The model under review builds one solid part; all positions refer to its coordinate system, in mm. Face numbers are marked on the shaded views. A direction names the side the tool comes from. Round coordinates to 2 decimals unless told otherwise and drop trailing zeros. Loops run counter-clockwise (first coordinate to the right, second up) from the corner with the lowest first, then second, coordinate; pieces in that order, holes last. Notation, with made-up numbers: (-16, 26) -> (36, 26) arc R14 cw to (36, 46) -> close; hole circle Ø4 at (82, 4). An arc over 180 degrees is marked (long way). Use CSV: the item, a comma, the result in double quotes. Start each with the question number.
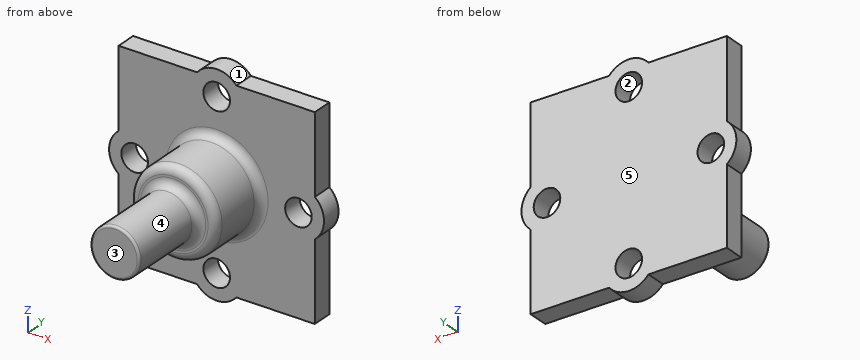
```python
from build123d import *

# Parameters (mm, degrees)
SKETCH1_R           = 3.25
BOSS_EXTRUDE1_DEPTH = 5
SKETCH2_W           = 32.64938716
SKETCH2_H           = 32.90693226
BOSS_EXTRUDE2_DEPTH = 5
SKETCH3_R           = 10.567193536
BOSS_EXTRUDE3_DEPTH = 15
SKETCH4_R           = 6
BOSS_EXTRUDE4_DEPTH = 20
FILLET1_R           = 2
FILLET2_R           = 0.56


with BuildPart() as part:
    # Sketch1 → Boss-Extrude1 (new body)
    with BuildSketch(Plane(origin=(0, 0, 0), x_dir=(1, 0, 0), z_dir=(0, 1, 0))):
        with BuildLine():
            Line((-24, -4.668943148), (-24, -24))
            Line((-24, -24), (-4.802343178, -24))
            ThreePointArc((-4.802343178, -24), (0, -26.25), (4.802343178, -24))
            Line((4.802343178, -24), (24, -24))
            Line((24, -24), (24, -4.802343178))
            ThreePointArc((24, -4.802343178), (26.25, 0), (24, 4.802343178))
            Line((24, 4.802343178), (24, 24))
            Line((24, 24), (4.802343178, 24))
            ThreePointArc((4.802343178, 24), (0, 26.25), (-4.802343178, 24))
            Line((-4.802343178, 24), (-24, 24))
            Line((-24, 24), (-24, 5.04363247))
            ThreePointArc((-24, 5.04363247), (-26.315667945, 0.187344661), (-24, -4.668943148))
        make_face()
        with Locations(Location((-20.065667945, 0.187344661, 0), (0, 0, 270))):
            Circle(SKETCH1_R, mode=Mode.SUBTRACT)
        with Locations(Location((0, 20, 0), (0, 0, 270))):
            Circle(SKETCH1_R, mode=Mode.SUBTRACT)
        with Locations(Location((20, 0, 0), (0, 0, 270))):
            Circle(SKETCH1_R, mode=Mode.SUBTRACT)
        with Locations(Location((0, -20, 0), (0, 0, 270))):
            Circle(SKETCH1_R, mode=Mode.SUBTRACT)
        with BuildLine():
            Line((-16, 16), (-4.802343178, 16))
            ThreePointArc((-4.802343178, 16), (0, 13.75), (4.802343178, 16))
            Line((4.802343178, 16), (16, 16))
            Line((16, 16), (16, 4.802343178))
            ThreePointArc((16, 4.802343178), (13.75, 0), (16, -4.802343178))
            Line((16, -4.802343178), (16, -16))
            Line((16, -16), (4.802343178, -16))
            ThreePointArc((4.802343178, -16), (0, -13.75), (-4.802343178, -16))
            Line((-4.802343178, -16), (-16, -16))
            Line((-16, -16), (-16, -4.559532645))
            ThreePointArc((-16, -4.559532645), (-13.815667945, 0.187344661), (-16, 4.934221967))
            Line((-16, 4.934221967), (-16, 16))
        make_face(mode=Mode.SUBTRACT)
    extrude(amount=BOSS_EXTRUDE1_DEPTH)

    # Sketch2 → Boss-Extrude2 (add)
    with BuildSketch(Plane.XZ):
        Rectangle(SKETCH2_W, SKETCH2_H)
    extrude(amount=-BOSS_EXTRUDE2_DEPTH)

    # Sketch3 → Boss-Extrude3 (add)
    with BuildSketch(Plane(origin=(0, 0, 0), x_dir=(-1, 0, 0), z_dir=(0, -1, 0))):
        with Locations(Location((0, 0, 0), (0, 0, 270))):
            Circle(SKETCH3_R)
    extrude(amount=BOSS_EXTRUDE3_DEPTH)

    # Sketch4 → Boss-Extrude4 (add)
    with BuildSketch(Plane(origin=(0, -15, 0), x_dir=(-1, 0, 0), z_dir=(0, -1, 0))):
        with Locations(Location((0, 0, 0), (0, 0, 90))):
            Circle(SKETCH4_R)
    extrude(amount=BOSS_EXTRUDE4_DEPTH)

    # Fillet1
    fillet1_edges = [part.edges().sort_by_distance(p)[0] for p in [
        (0, 0, -10.567193536),
        (0, -15, -10.567193536),
        (0, -15, 6),
    ]]
    fillet(fillet1_edges, radius=FILLET1_R)

    # Fillet2
    fillet2_edges = [part.edges().sort_by_distance(p)[0] for p in [
        (0, -35, 6),
    ]]
    fillet(fillet2_edges, radius=FILLET2_R)


solid = part.part
```
1. Take a section at D-D, the plane z = 0. Give the boundary of the cut face in (x, y).
2. For line 1 along X through (y, z) = (2.7, 0); line 2 along X through (y, z) = (3, 20); line 3 along Y through (x, z) = (2.5, -24), list the stretches that pass through material, from the lowest coordinate up. Write a range as from..to.
3. Clearance check with flat-ended pins moving along their axes: P1, Ø2.5, axis at y = 1.5, z = -10, coming from the +X side; P2, Ø1.5, axis at x = -19, y = 1.5, coming from the -Z side; P3, Ø4, axis at x = 20, z = 0, coming from the +Y side; P4, Ø5, axis at x = -10, z = -7.5, coming from the -Y side. State where each tip first meets the part, or that it passes through.
4. For the marked faces 4 and 5, list the 3-axis set-ups (+Z, -Z, +X, -X, +Y, -Y) from which the entire face can be reached by the end or side of a thin tool; tool diameter is ignored.
5. Take a section at A-A, the plane x = 0. Give the boundary of the cut face in (y, z), then the cut area to 3 significant figures.
6. Take a section at B-B, the plane x = 20. Give the boundary of the cut face in (y, z), then the cut area to 4 significant figures.
7. Take a section at C-C, the plane z = -20. Give the boundary of the cut face in (x, y).
8. The part is to be moulded in two halves that separate along Z. For the marked faces 1, 2 and 3, say which applies: pulls with the +Z half, pulls with the -Z half, needs draft (parallel to the pull), parting line crosses it, or undercut.
Results:
1,outline,"(-26.31, 0) -> (-23.31, 0) -> (-23.31, 5) -> (-26.31, 5) -> close; (-16.82, 0) -> (-12.57, 0) arc R2 cw to (-10.57, -2) -> (-10.57, -13) arc R2 ccw to (-8.57, -15) -> (-8, -15) arc R2 cw to (-6, -17) -> (-6, -34.44) arc R0.56 ccw to (-5.44, -35) -> (5.44, -35) arc R0.56 ccw to (6, -34.44) -> (6, -17) arc R2 cw to (8, -15) -> (8.57, -15) arc R2 ccw to (10.57, -13) -> (10.57, -2) arc R2 cw to (12.57, 0) -> (16.75, 0) -> (16.75, 5) -> (-16.82, 5) -> close; (23.25, 0) -> (26.25, 0) -> (26.25, 5) -> (23.25, 5) -> close"
2,line 1,"-26.31..-23.31, -16.82..16.75, 23.25..26.25"
2,line 2,"-24..-3.25, 3.25..24"
2,line 3,"0..5"
3,P1,"x = 24"
3,P2,"z = -24"
3,P3,"through"
3,P4,"y = -14.4"
4,face 4,"-Y"
4,face 5,"+Z, -Z, +X, -X, +Y"
5,outline,"(-35, -5.44) arc R0.56 ccw to (-34.44, -6) -> (-17, -6) arc R2 cw to (-15, -8) -> (-15, -8.57) arc R2 ccw to (-13, -10.57) -> (-2, -10.57) arc R2 cw to (0, -12.57) -> (0, -16.75) -> (5, -16.75) -> (5, 16.75) -> (0, 16.75) -> (0, 12.57) arc R2 cw to (-2, 10.57) -> (-13, 10.57) arc R2 ccw to (-15, 8.57) -> (-15, 8) arc R2 cw to (-17, 6) -> (-34.44, 6) arc R0.56 ccw to (-35, 5.44) -> close; (0, -26.25) -> (5, -26.25) -> (5, -23.25) -> (0, -23.25) -> close; (0, 23.25) -> (5, 23.25) -> (5, 26.25) -> (0, 26.25) -> close"
5,area,"756 mm²"
6,outline,"(0, -24) -> (5, -24) -> (5, -3.25) -> (0, -3.25) -> close; (0, 3.25) -> (5, 3.25) -> (5, 24) -> (0, 24) -> close"
6,area,"207.5 mm²"
7,outline,"(-24, 0) -> (-3.25, 0) -> (-3.25, 5) -> (-24, 5) -> close; (3.25, 0) -> (24, 0) -> (24, 5) -> (3.25, 5) -> close"
8,face 1,"pulls with the +Z half"
8,face 2,"undercut"
8,face 3,"needs draft"
